Geometry: final body of the model. Coordinates: model frame, mm. Face numbers are marked on the shaded views. A direction names the side the tool comes from. Give positions to 0.01 mm unless a question says otherwise; leave off trailing zeros. Loops run counter-clockwise (first coordinate to the right, second up) from the corner with the lowest first, then second, coordinate; pieces in that order, holes last. Notation, with made-up numbers: M 65.5,-7.75 L 119.5,-7.75 A23 cw 119.5,2.25 Z; hole C 41,-31 d8. An arc over 180 degrees is marked long. Put each result on its own line as item: value.
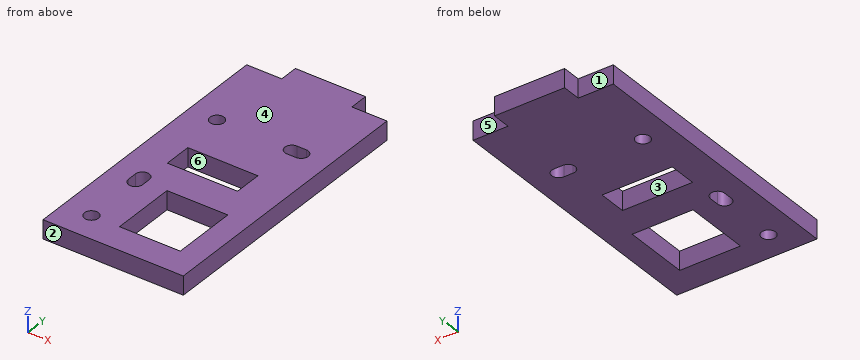
```python
from build123d import *

# Parameters (mm, degrees)
SKETCH1_R           = 1.5
SKETCH1_W           = 13
SKETCH1_H           = 14
SKETCH1_W_2         = 15
SKETCH1_H_2         = 6
BOSS_EXTRUDE1_DEPTH = 4


with BuildPart() as part:
    # Sketch1 → Boss-Extrude1 (new body)
    with BuildSketch(Plane.XY):
        Polygon((0, 0), (30, 0), (30, 60), (22.5, 60), (22.5, 64), (7.5, 64), (7.5, 60), (0, 60), align=None)
        with Locations((6, 6)):
            Circle(SKETCH1_R, mode=Mode.SUBTRACT)
        with Locations((6, 43)):
            Circle(SKETCH1_R, mode=Mode.SUBTRACT)
        with Locations((18.5, 13)):
            Rectangle(SKETCH1_W, SKETCH1_H, mode=Mode.SUBTRACT)
        with Locations((14.5, 30)):
            Rectangle(SKETCH1_W_2, SKETCH1_H_2, mode=Mode.SUBTRACT)
        with BuildLine():
            Line((7.5, 21), (7.5, 19))
            ThreePointArc((7.5, 19), (6, 17.5), (4.5, 19))
            Line((4.5, 19), (4.5, 21))
            ThreePointArc((4.5, 21), (6, 22.5), (7.5, 21))
        make_face(mode=Mode.SUBTRACT)
        with BuildLine():
            Line((22, 44.5), (24, 44.5))
            ThreePointArc((24, 44.5), (25.5, 43), (24, 41.5))
            Line((24, 41.5), (22, 41.5))
            ThreePointArc((22, 41.5), (20.5, 43), (22, 44.5))
        make_face(mode=Mode.SUBTRACT)
    extrude(amount=BOSS_EXTRUDE1_DEPTH)


solid = part.part
```
Item 1: Pin query (flat end, axial travel): pin 1 Ø1.2 at (y, z) = (62.5, 1.5) entering from +X; pin 2 Ø3.5 at (x, y) = (6, 6) entering from -Z; pin 3 Ø1.2 at (x, z) = (5, 2.5) entering from +Y. Return the tip coordinate at first contact, or that it passes through.
Output values:
pin 1: x = 22.5
pin 2: z = 0
pin 3: y = 60
Item 2: Section A-A on x = 9. Output: boundary loops of the cut face in (y, z).
Output values:
outline: M 0,0 L 27,0 L 27,4 L 0,4 Z; M 33,0 L 64,0 L 64,4 L 33,4 Z
Item 3: Section B-B on x = 6. Output: boundary loops of the cut face in (y, z).
Output values:
outline: M 0,0 L 4.5,0 L 4.5,4 L 0,4 Z; M 7.5,0 L 17.5,0 L 17.5,4 L 7.5,4 Z; M 22.5,0 L 41.5,0 L 41.5,4 L 22.5,4 Z; M 44.5,0 L 60,0 L 60,4 L 44.5,4 Z
Item 4: Mould query, pull axis Y, two halves, no side actions, for the marked faces 1, 2 and 3. Classes: pulls with the +Y half, pulls with the -Y half, needs draft (parallel to the pull), parting line crosses it, or undercut.
Output values:
face 1: pulls with the +Y half
face 2: pulls with the -Y half
face 3: undercut
Item 5: Set-up query: the marked faces 4, 5 and 6. Return all of +Z, -Z, +X, -X, +Y, -Y with unobstructed straight access to the full face (end or side cutting, diameter ignored); none if empty.
Output values:
face 4: +Z, +X, -X, +Y, -Y
face 5: +Z, -Z, +X, +Y
face 6: +Z, -Z
Item 6: Section C-C on y = 43. Output: boundary loops of the cut face in (x, z), then the cut area to 3 significant figures.
Output values:
outline: M 0,0 L 4.5,0 L 4.5,4 L 0,4 Z; M 7.5,0 L 20.5,0 L 20.5,4 L 7.5,4 Z; M 25.5,0 L 30,0 L 30,4 L 25.5,4 Z
area: 88.0 mm²
Item 7: Line query: probe 1 along Y at (x, z) = (6, 2.2); probe 2 along Y at (x, z) = (16.5, 2.4); probe 3 along X at (y, z) = (8, 2.35). Output: solid intervals per line, ascending. Write a range as [from, to].
Output values:
probe 1: [0, 4.5], [7.5, 17.5], [22.5, 41.5], [44.5, 60]
probe 2: [0, 6], [20, 27], [33, 64]
probe 3: [0, 12], [25, 30]
Item 8: Section D-D on z = 3.05. Output: boundary loops of the cut face in (x, y).
Output values:
outline: M 0,0 L 30,0 L 30,60 L 22.5,60 L 22.5,64 L 7.5,64 L 7.5,60 L 0,60 Z; hole C 6,6 d3; hole M 4.5,19 A1.5 ccw 7.5,19 L 7.5,21 A1.5 ccw 4.5,21 Z; hole C 6,43 d3; hole M 7,27 L 22,27 L 22,33 L 7,33 Z; hole M 12,6 L 25,6 L 25,20 L 12,20 Z; hole M 22,41.5 L 24,41.5 A1.5 ccw 24,44.5 L 22,44.5 A1.5 ccw Z
